Read the model definition and answer for the solid it produces. Units are mm, in the model's axes. Face numbers are marked on the shaded views. Coordinates: 2 decimals unless noted, no trailing zeros. Loops run counter-clockwise (first coordinate to the right, second up) from the corner with the lowest first, then second, coordinate; pieces in that order, holes last. Notation, with made-up numbers: M 9.5,-27.5 L 18.5,-27.5 A17 cw 18.5,-16.5 Z; hole C 62.25,67.25 d9. An arc over 180 degrees is marked long. Put each result on its own line as item: value.
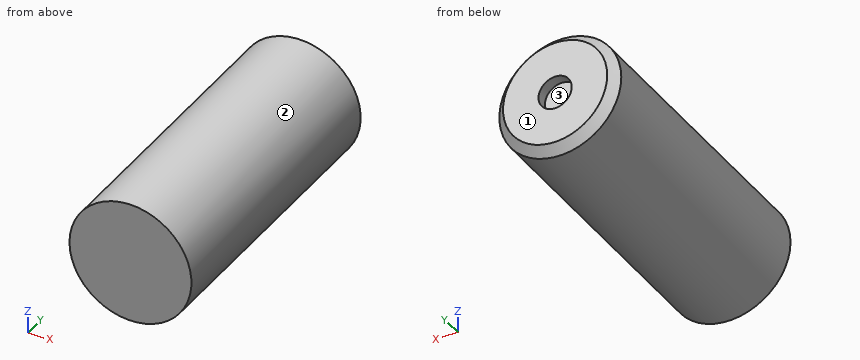
Autodesk Inventor part; units mm, degrees
ref_plane "YZ Plane" through (0, 0, 0) normal (1, 0, 0) x (0, 1, 0)
ref_plane "XZ Plane" through (0, 0, 0) normal (0, 1, 0) x (-1, 0, 0)
ref_plane "XY Plane" through (0, 0, 0) normal (0, 0, 1) x (1, 0, 0)
sketch "Sketch1" plane through (0, 0, 0) normal (0, 1, 0) x (-1, 0, 0)
  circle A0 centre (0, 0) radius 2.75
  dimension "d0" = 5.5
extrude "Extrusion1" add sketch "Sketch1" along normal blind 13.447
chamfer "Chamfer1" distance 0.4 angle 45 1 edges at (2.75, 13.447, 0)
sketch "Sketch2" plane through (0, 13.447, 0) normal (0, 1, 0) x (1, 0, 0)
  circle A0 centre (0, 0) radius 2.35
  circle A1 centre (0, 0) radius 0.75
  dimension "d6" = 1.5
extrude "Extrusion2" cut sketch "Sketch2" against normal blind 0.5 contours A1
properties part number "controller_push_button" material "ABS Plastic"
1) Find section A-A, the plane y = 3. Write down the section's boundary in (x, z).
Answer list:
outline: C 0,0 d5.5
2) Given pin 1 Ø1.5 at (x, y) = (-1, 5.5) entering from -Z; pin 2 Ø0.9 at (x, z) = (0, 0) entering from +Y, each flat-ended and moving along its own axis, determine where each tip first touches the part or whether it passes through.
Answer list:
pin 1: stops at z = -2.74
pin 2: stops at y = 12.95
3) Straight lines are drawn through the part: line 1 (X direction, y = 13.1, z = 0); line 2 (Z direction, x = 0, y = 13.35); line 3 (Z direction, x = 0, y = 13.25). For each, find the intervals that lie inside material, in ascending order. Write a range as [from, to].
Answer list:
line 1: x = [-2.7, -0.75], [0.75, 2.7]
line 2: z = [-2.45, -0.75], [0.75, 2.45]
line 3: z = [-2.55, -0.75], [0.75, 2.55]
4) Determine the mould class of the marked faces 1, 2 and 3 for opening direction X: released by +X, released by -X, zero draft, split by the parting line, or undercut.
Answer list:
face 1: zero draft
face 2: split by the parting line
face 3: undercut
